from build123d import *

# Parameters (mm, degrees)
F0_W     = 76.2
F0_H     = 25.4
F1_DEPTH = 12.7
F3_DEPTH = 33.02
F4_R     = 10.16
F5_DEPTH = 35.56
F6_R     = 6.35
F7_DEPTH = 38.1


with BuildPart() as f1:
    # F0 (on Front) → F1 (new body, symmetric)
    with BuildSketch(Plane.XZ):
        Rectangle(F0_W, F0_H)
    extrude(amount=F1_DEPTH, both=True)

    # F2 (on face) → F3 (join)
    with BuildSketch(Plane(origin=(0, 0, -12.7), x_dir=(1, 0, 0), z_dir=(0, 0, -1))):
        with BuildLine():
            ThreePointArc((0, -12.7), (8.980256, -8.980256), (12.7, 0))
            ThreePointArc((12.7, 0), (8.980256, 8.980256), (0, 12.7))
            ThreePointArc((0, 12.7), (-12.7, 0), (0, -12.7))
        make_face()
    extrude(amount=F3_DEPTH)

    # F4 (on face) → F5 (join)
    with BuildSketch(Plane.YZ.offset(38.1)):
        Circle(F4_R)
    extrude(amount=F5_DEPTH)

    # F6 (on face) → F7 (join)
    with BuildSketch(Plane.YZ.offset(73.66)):
        Circle(F6_R)
    extrude(amount=F7_DEPTH)


solid = f1.part
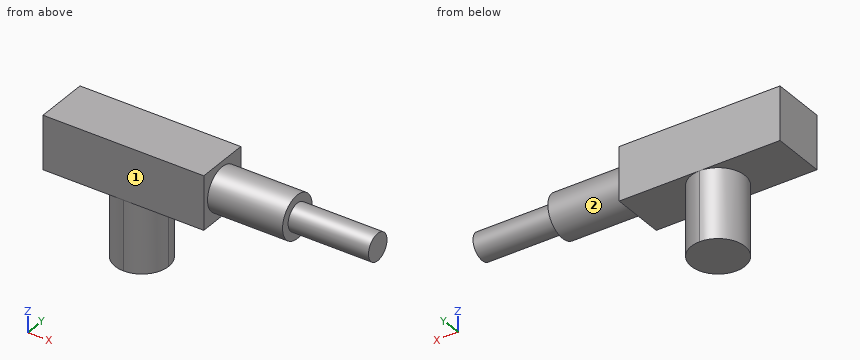
Verification items for the finished model (mm, model axes). Face numbers are marked on the shaded views. A direction names the side the tool comes from. Round coordinates to 2 decimals unless told otherwise and drop trailing zeros. Order: outer loops, then holes, each group sorted by start corner. A loop starts at its lowest first (then second) coordinate and runs counter-clockwise, first axis right, second up. Notation, with made-up numbers: (86, 28.25) -> (92, 28.25) arc R27 cw to (92, 54.25) -> close; hole circle Ø7 at (-25, 42.5). An arc over 180 degrees is marked (long way). Put each result on its own line as item: value.
1) Section check D-D (x = 18). Record the cut outline in (y, z), then the cut area to 3 significant figures.
Final values:
outline: (-12.7, -12.7) -> (12.7, -12.7) -> (12.7, 12.7) -> (-12.7, 12.7) -> close
area: 645 mm^2
2) Section check C-C (x = 46.5). Record the cut outline in (y, z), then the cut area to 3 significant figures.
Final values:
outline: circle Ø20.32 at (0, 0)
area: 324 mm^2
3) Set-up check for the marked faces 1 and 2: record each of +Z, -Z, +X, -X, +Y, -Y from which the full face is reachable in a straight line by a thin tool's end or side.
Final values:
face 1: +Z, -Z, +X, -X, -Y
face 2: +X
4) Material ranges on line 1 (X direction, y = 0.75, z = -34); line 2 (Z direction, x = 33.5, y = 0.5); line 3 (X direction, y = -2.5, z = 9.5), recorded low to high.
Final values:
line 1: x = -12.68 to 12.68
line 2: z = -12.7 to 12.7
line 3: x = -38.1 to 73.66
5) Section check A-A (y = 8). Record the cut outline in (x, z).
Final values:
outline: (-38.1, -12.7) -> (-9.86, -12.7) -> (-9.86, -45.72) -> (9.86, -45.72) -> (9.86, -12.7) -> (38.1, -12.7) -> (38.1, -6.26) -> (73.66, -6.26) -> (73.66, 6.26) -> (38.1, 6.26) -> (38.1, 12.7) -> (-38.1, 12.7) -> close
6) Section check B-B (z = 0). Record the cut outline in (x, y).
Final values:
outline: (-38.1, -12.7) -> (38.1, -12.7) -> (38.1, -10.16) -> (73.66, -10.16) -> (73.66, -6.35) -> (111.76, -6.35) -> (111.76, 6.35) -> (73.66, 6.35) -> (73.66, 10.16) -> (38.1, 10.16) -> (38.1, 12.7) -> (-38.1, 12.7) -> close
7) Depth check by flat-ended pin: pin 1 (10 mm diameter, centred on x = 57, y = 8, fed in from -Z); pin 2 (8 mm diameter, centred on x = -9, z = -23.5, fed in from +Y); pin 3 (10 mm diameter, centred on y = -6, z = -26.5, fed in from -X). Enter the tip coordinate at first touch or a pass-through.
Final values:
pin 1: stops at z = -9.71
pin 2: stops at y = 11.67
pin 3: stops at x = -12.66
